The listing builds one solid part. Answer for the finished solid, in the listing's coordinates (mm). Give positions to 0.01 mm unless a question says otherwise; leave off trailing zeros. Order: outer loops, then holes, each group sorted by start corner. A loop starts at its lowest first (then second) coordinate and runs counter-clockwise, first axis right, second up. Notation, with made-up numbers: (-7, -26) - (-1, -26) arc R16 cw to (-1, -15) - close; hole circle Ø5 at (-24.75, 28.25). An arc over 180 degrees is marked (long way). Answer in a Markdown table with one row per item.
from build123d import *

# Parameters (mm, degrees)
SKETCH1_R           = 12.7
BOSS_EXTRUDE1_DEPTH = 3.175
SKETCH3_R           = 12.7
CUT_EXTRUDE1_DEPTH  = 4.175
SKETCH4_W           = 50.8
SKETCH4_H           = 228.6
CUT_EXTRUDE2_DEPTH  = 4.175
BOSS_EXTRUDE2_DEPTH = 3.175
CUT_EXTRUDE3_DEPTH  = 4.175
FILLET1_R           = 9.525


with BuildPart() as part:
    # Sketch1 → Boss-Extrude1 (new body)
    with BuildSketch(Plane(origin=(0, 0, 0), x_dir=(0, 0, -1), z_dir=(1, 0, 0))):
        Polygon((-228.6, 25.4), (228.6, 25.4), (228.6, -254), (177.8, -254), (177.8, -25.4), (-177.8, -25.4), (-177.8, -254), (-228.6, -254), align=None)
        Circle(SKETCH1_R, mode=Mode.SUBTRACT)
    extrude(amount=BOSS_EXTRUDE1_DEPTH)

    # Sketch3 → Cut-Extrude1 (cut, through all)
    with BuildSketch(Plane(origin=(3.175, 0, 0), x_dir=(0, 0, -1), z_dir=(1, 0, 0))):
        with Locations((-203.2, -228.6)):
            Circle(SKETCH3_R)
        with Locations((203.2, -228.6)):
            Circle(SKETCH3_R)
    extrude(amount=-CUT_EXTRUDE1_DEPTH, mode=Mode.SUBTRACT)

    # Sketch4 → Cut-Extrude2 (cut, through all)
    with BuildSketch(Plane(origin=(3.175, 0, 0), x_dir=(0, 0, -1), z_dir=(1, 0, 0))):
        with Locations((-203.2, -139.7)):
            Rectangle(SKETCH4_W, SKETCH4_H)
    extrude(amount=-CUT_EXTRUDE2_DEPTH, mode=Mode.SUBTRACT)

    # Sketch5 → Boss-Extrude2 (add)
    with BuildSketch(Plane(origin=(3.175, 0, 0), x_dir=(0, 0, -1), z_dir=(1, 0, 0))):
        Polygon((50.8, -25.4), (177.8, -152.4), (177.8, -25.4), align=None)
    extrude(amount=-BOSS_EXTRUDE2_DEPTH)

    # Sketch6 → Cut-Extrude3 (cut, through all)
    with BuildSketch(Plane(origin=(3.175, 0, 0), x_dir=(0, 0, -1), z_dir=(1, 0, 0))):
        Polygon((71.842048969, 25.4), (228.6, -131.357951031), (228.6, 25.4), align=None)
    extrude(amount=-CUT_EXTRUDE3_DEPTH, mode=Mode.SUBTRACT)

    # Fillet1
    fillet1_edges = [part.edges().sort_by_distance(p)[0] for p in [
        (1.5875, 25.4, 228.6),
        (1.5875, -254, -228.6),
        (1.5875, -254, -177.8),
        (1.5875, -25.4, 228.6),
        (1.5875, -25.4, -50.8),
        (1.5875, -152.4, -177.8),
        (1.5875, 25.4, -71.842048969),
        (1.5875, -131.357951031, -228.6),
    ]]
    fillet(fillet1_edges, radius=FILLET1_R)


solid = part.part
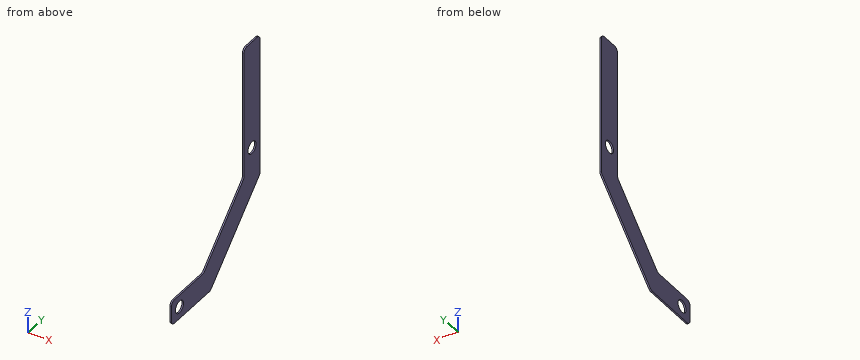
Item 1: Find section C-C on z = 0. Write down the section's boundary in (x, y) (3 decimals).
Answer block:
| item | result |
|---|---|
| outline | (0, -25.4) - (3.175, -25.4) - (3.175, -12.7) - (0, -12.7) - close; (0, 12.7) - (3.175, 12.7) - (3.175, 25.4) - (0, 25.4) - close |
Item 2: Find section D-D on y = -176. Write down the section's boundary in (x, z) (3 decimals).
Answer block:
| item | result |
|---|---|
| outline | (0, -228.6) - (3.175, -228.6) - (3.175, -177.8) - (0, -177.8) - close |
Item 3: Find section B-B on x = 2.5. Write down the section's boundary in (y, z) (3 decimals), then the cut area to 3 significant figures.
Answer block:
| item | result |
|---|---|
| outline | (-254, -219.075) arc R9.525 ccw to (-244.475, -228.6) - (-135.303, -228.6) arc R9.525 ccw to (-128.568, -225.81) - (22.61, -74.632) arc R9.525 ccw to (25.4, -67.897) - (25.4, 219.075) arc R9.525 ccw to (15.875, 228.6) - (-15.875, 228.6) arc R9.525 ccw to (-25.4, 219.075) - (-25.4, -46.855) arc R9.525 cw to (-28.19, -53.59) - (-149.61, -175.01) arc R9.525 cw to (-156.345, -177.8) - (-244.475, -177.8) arc R9.525 ccw to (-254, -187.325) - close; hole circle Ø25.4 at (-228.6, -203.2); hole circle Ø25.4 at (0, 0) |
| area | 29,500 mm² |
Item 4: Find section A-A on y = -228.6. Write down the section's boundary in (x, z) (3 decimals), then the cut area to 3 significant figures.
Answer block:
| item | result |
|---|---|
| outline | (0, -228.6) - (3.175, -228.6) - (3.175, -215.9) - (0, -215.9) - close; (0, -190.5) - (3.175, -190.5) - (3.175, -177.8) - (0, -177.8) - close |
| area | 80.6 mm² |
Item 5: Each of these flat-tipped pins is pushed along its axis until it touches: P1, Ø1, axis at x = 1.5, y = -210, coming from the +Z side; P2, Ø15, axis at y = -228.6, z = -203.2, coming from the -X side. Where does it stop, or does it pass through?
Answer block:
| item | result |
|---|---|
| P1 | z = -177.8 |
| P2 | through |
Item 6: Consider line 1 (Y direction, x = 0.8, z = 146); line 2 (Y direction, x = 1.55, z = -203.2); line 3 (Z direction, x = 0.65, y = -35). Determine where each line is inside the solid, lowest interval first.
Answer block:
| item | result |
|---|---|
| line 1 | -25.4 to 25.4 |
| line 2 | -254 to -241.3, -215.9 to -105.96 |
| line 3 | -132.24 to -60.4 |
